CAD build for the part. Positions are in the model's coordinates, mm. Face numbers are marked on the shaded views. A direction names the side the tool comes from. Round coordinates to 2 decimals unless told otherwise and drop trailing zeros. Loops run counter-clockwise (first coordinate to the right, second up) from the corner with the lowest first, then second, coordinate; pieces in that order, holes last. Notation, with made-up numbers: (60, 38) -> (86, 38) arc R20 cw to (86, 68) -> close; hole circle Ø6 at (67.25, 31.5). An arc over 180 degrees is marked (long way). Answer as CSV lines item,"result".
```python
from build123d import *

# Parameters (mm, degrees)
PAD_DEPTH       = 22.5
POCKET_DEPTH    = 20
SKETCH002_R     = 1.6
POCKET001_DEPTH = 5
SKETCH003_R     = 1.8
POCKET002_DEPTH = 5
CHAMFER001_SIZE = 4
CHAMFER_SIZE    = 1
POCKET003_DEPTH = 5.5
SKETCH005_W     = 8
SKETCH005_H     = 29
POCKET004_DEPTH = 0.2


with BuildPart() as part:
    # Sketch → Pad (new body, symmetric)
    with BuildSketch(Plane.XZ):
        Polygon((0, 0), (8.559569, 0), (8.559569, 1.2), (0.559569, 1.2), (-5.512797, 8.436764), (-5.512797, 23), (-6.712797, 23), (-6.712797, 8), align=None)
    extrude(amount=PAD_DEPTH, both=True)

    # Sketch001 (on Face7 of Pad) → Pocket (cut)
    with BuildSketch(Plane(origin=(-6.712797, 0, 0), x_dir=(0, 0, -1), z_dir=(-1, 0, 0))):
        Polygon((-8, -22.5), (0, -12.965971), (0, -23.5), (-8, -23.5), align=None)
        Polygon((-8, 22.5), (0, 12.965971), (0, 23.5), (-8, 23.5), align=None)
    extrude(amount=-POCKET_DEPTH, mode=Mode.SUBTRACT)

    # Sketch002 (on Face6 of Pocket) → Pocket001 (cut)
    with BuildSketch(Plane(origin=(0, 0, 1.2), x_dir=(-1, 0, 0), z_dir=(0, 0, 1))):
        with Locations((-4.5, 10)):
            Circle(SKETCH002_R)
        with Locations((-4.5, -10)):
            Circle(SKETCH002_R)
        Polygon((-9.5, -9.5), (-4.5, -4.5), (-4.5, 4.5), (-9.5, 9.5), align=None)
    extrude(amount=-POCKET001_DEPTH, mode=Mode.SUBTRACT)

    # Sketch003 (on Face16 of Pocket001) → Pocket002 (cut)
    with BuildSketch(Plane(origin=(-6.712797, 0, 0), x_dir=(0, 0, -1), z_dir=(-1, 0, 0))):
        with Locations((-16, 18)):
            Circle(SKETCH003_R)
        with Locations((-16, -18)):
            Circle(SKETCH003_R)
    extrude(amount=-POCKET002_DEPTH, mode=Mode.SUBTRACT)

    # Chamfer001
    chamfer001_edges = [part.edges().sort_by_distance(p)[0] for p in [
        (-6.112797, -22.5, 23),
        (-6.112797, 22.5, 23),
    ]]
    chamfer(chamfer001_edges, length=CHAMFER001_SIZE)

    # Chamfer
    chamfer_edges = [part.edges().sort_by_distance(p)[0] for p in [
        (8.559569, -13.681023, 0.6),
        (8.559569, 13.681023, 0.6),
    ]]
    chamfer(chamfer_edges, length=CHAMFER_SIZE)

    # Sketch004 (on Face19 of Chamfer) → Pocket003 (cut, symmetric)
    with BuildSketch(Plane(origin=(-5.512797, 0, 0), x_dir=(0, 0, 1), z_dir=(1, 0, 0))):
        Polygon((1.4, 6.5), (1.4, -6.5), (3, -11.5), (7, -11.5), (7, 11.5), (3, 11.5), align=None)
    extrude(amount=POCKET003_DEPTH, both=True, mode=Mode.SUBTRACT)

    # Sketch005 (on Face5 of Pocket003) → Pocket004 (cut)
    with BuildSketch(Plane(origin=(0, 0, 1.2), x_dir=(-1, 0, 0), z_dir=(0, 0, 1))):
        with Locations((-5, 0)):
            Rectangle(SKETCH005_W, SKETCH005_H)
    extrude(amount=-POCKET004_DEPTH, mode=Mode.SUBTRACT)


solid = part.part
```
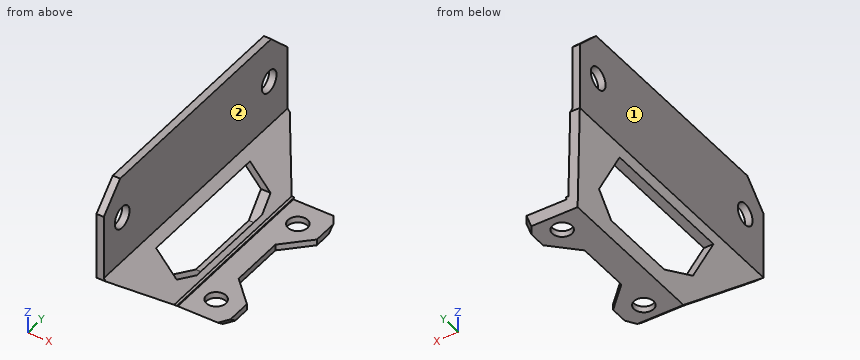
Q1. Slice it at B-B, the plane z = 15.25. Give the cut face in (x, y), and give its area (3 significant figures).
Results:
outline,"(-6.71, -22.5) -> (-5.51, -22.5) -> (-5.51, -19.64) -> (-6.71, -19.64) -> close; (-6.71, -16.36) -> (-5.51, -16.36) -> (-5.51, 16.36) -> (-6.71, 16.36) -> close; (-6.71, 19.64) -> (-5.51, 19.64) -> (-5.51, 22.5) -> (-6.71, 22.5) -> close"
area,"46.1 mm2"
Q2. Slice it at A-A, the plane y = -0.5. Give the cut face in (x, z).
Results:
outline,"(-6.71, 8) -> (-5.87, 7) -> (-4.31, 7) -> (-5.51, 8.44) -> (-5.51, 23) -> (-6.71, 23) -> close; (-1.17, 1.4) -> (0, 0) -> (4.5, 0) -> (4.5, 1) -> (1, 1) -> (1, 1.2) -> (0.56, 1.2) -> (-0.01, 1.88) -> (-0.01, 1.4) -> close"
Q3. Slice it at D-D, the plane z = 11.5. Give the cut face in (x, y), and give its area (3 significant figures).
Results:
outline,"(-6.71, -22.5) -> (-5.51, -22.5) -> (-5.51, 22.5) -> (-6.71, 22.5) -> close"
area,"54.0 mm2"
Q4. Tool access for the marked faces 1 and 2: list every direction of +Z, -Z, +X, -X, +Y, -Y with a clear straight run to the whole face (end or side of a thin tool).
Results:
face 1,"+Z, -Z, -X, +Y, -Y"
face 2,"+Z, +X, +Y, -Y"
Q5. Probe L1, parallel to Y at x = -6.35, z = 16; L2, parallel to X at y = 14, z = 9; L3, parallel to Z at x = -5.75, y = -3. List the from-to ranges inside material, lowest first. Write a range as [from, to].
Results:
L1,"[-22.5, -19.8], [-16.2, 16.2], [19.8, 22.5]"
L2,"[-6.71, -5.51]"
L3,"[7, 23]"
Q6. Drop flat-ended pins along their axis: pin 1 Ø1 at (x, y) = (-3.5, 10.5) entering from +Z; pin 2 Ø1.5 at (x, y) = (-1.5, -10.5) entering from -Z; pin 3 Ø1.1 at (y, z) = (1.5, 0.5) entering from +X; pin 4 Ø1 at (y, z) = (-11.5, 15.5) entering from +X. Give the stop position or say it passes through.
Results:
pin 1,"through"
pin 2,"z = 0.89"
pin 3,"x = 4.5"
pin 4,"x = -5.51"
Q7. Slice it at C-C, the plane y = 10. Give the cut face in (x, z), and give its area (3 significant figures).
Results:
outline,"(-6.71, 8) -> (-5.87, 7) -> (-4.31, 7) -> (-5.51, 8.44) -> (-5.51, 23) -> (-6.71, 23) -> close; (-2.11, 2.52) -> (0, 0) -> (2.9, 0) -> (2.9, 1) -> (1, 1) -> (1, 1.2) -> (0.56, 1.2) -> (-0.55, 2.52) -> close; (6.1, 0) -> (8.56, 0) -> (8.56, 1) -> (6.1, 1) -> close"
area,"27.9 mm2"
